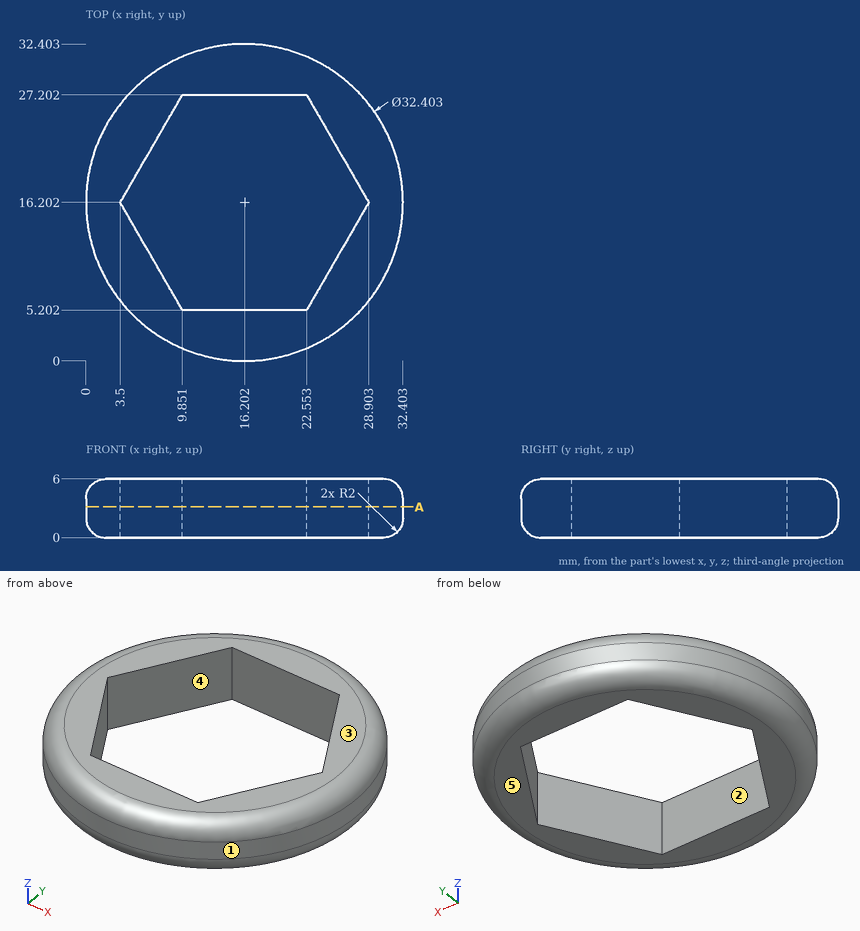
Geometry check sheet. Reference: drawing and pictorial views, mm from the part's lowest x, y, z. A direction names the side the tool comes from. Give positions to 0.01 mm unless a question says otherwise; leave off trailing zeros. Loops run counter-clockwise (first coordinate to the right, second up) from the corner with the lowest first, then second, coordinate; pieces in that order, holes last.
1. Thickness scan on line 1 (Y direction, x = 5, z = 1.95) (1 decimal); line 2 (X direction, y = 12, z = 0.3) (1 decimal); line 3 (Y direction, x = 15.5, z = 2.55) (1 decimal). Record the ranges inside material, lowest first.
2. Mould release check, pull along X, two halves, no side actions. Record for the marked faces 1, 2 and 3: released by +X, released by -X, zero draft, split by the parting line, or undercut.
3. Section check A-A, the plane z = 3.15. Enter the section's corners in (x, y).
4. Set-up check for the marked faces 4 and 5: record each of +Z, -Z, +X, -X, +Y, -Y from which the full face is reachable in a straight line by a thin tool's end or side.
5. Go/stop test with flat-tipped pins: pin 1 Ø1 at (y, z) = (24, 3.5) entering from -X; pin 2 Ø1 at (x, z) = (19.5, 2) entering from +Y; pin 3 Ø6 at (x, y) = (18, 23.5) entering from +Z; pin 4 Ø3 at (x, z) = (29, 2) entering from -Y. Record where each tip stops, or that it passes through.
Geometry says:
1. line 1: y = 4.5 to 13.6, 18.8 to 27.9
1. line 2: x = 1.5 to 5.9, 26.5 to 30.9
1. line 3: y = 0 to 5.2, 27.2 to 32.4
2. face 1: split by the parting line
2. face 2: undercut
2. face 3: zero draft
3. outline: circle Ø32.4 at (16.2, 16.2); hole (3.5, 16.2) - (9.85, 5.2) - (22.55, 5.2) - (28.9, 16.2) - (22.55, 27.2) - (9.85, 27.2) - close
4. face 4: +Z, -Z
4. face 5: -Z, +X, -X, +Y, -Y
5. pin 1: stops at x = 1.74
5. pin 2: stops at y = 32.16
5. pin 3: passes through
5. pin 4: stops at y = 4.59
